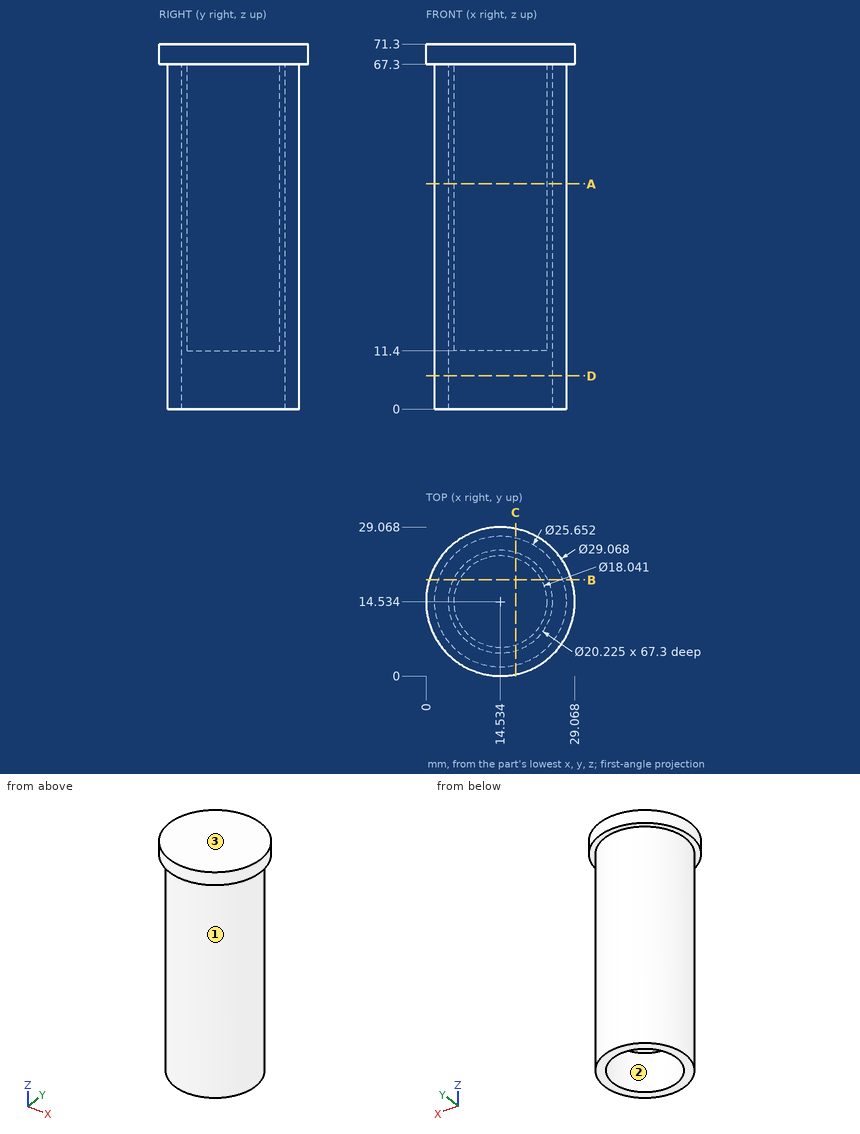
Design review of the part shown in the three views and the two pictorial views. Dimensions are in mm from the part's minimum x, y and z. Coordinates: 2 decimals unless noted, no trailing zeros. Order: outer loops, then holes, each group sorted by start corner. A loop starts at its lowest first (then second) coordinate and runs counter-clockwise, first axis right, second up. Notation, with made-up numbers: (38.5, 77) - (46.5, 77) arc R24 cw to (46.5, 91) - close; hole circle Ø6 at (5, -6). An arc over 180 degrees is marked (long way). Answer as CSV lines item,"result". Start each with the question number.
1) To check wall thickness, follow line 1 along X through (y, z) = (11.5, 13.5) (1 decimal); line 2 along Y through (x, z) = (16.25, 59) (1 decimal); line 3 along Y through (x, z) = (20.5, 53). State the ranges of each line that lie inside material, in increasing order. Write a range as [from, to].
2) Draft analysis for pull direction Y (two halves, no side actions). For the marked faces 1, 2 and 3, state which applies: +Y half, -Y half, draft (parallel to the pull), parting line (faces both ways), or undercut.
3) Add section C-C (x = 17.5). State the section outline as (y, z) points (1 decimal), then the cut area to 3 significant figures.
4) Add section D-D (z = 6.5). State the section outline as (x, y) points (1 decimal).
5) Add section A-A (z = 44). State the section outline as (x, y) points (1 decimal).
6) Add section B-B (y = 18.75). State the section outline as (x, z) points (1 decimal), then the cut area to 3 significant figures.
7) Insertion check: P1, Ø1, axis at x = 15, z = 31, coming from the +Y side; P2, Ø1.5, axis at x = 23, z = 52, coming from the +Y side; P3, Ø6, axis at x = 16.5, y = 10.5, coming from the -Z side. Each pin has a flat end and moves straight along its axis. Give the tip position at first contact, or say it passes through.
Result:
1,line 1,"[2.1, 4.9], [6, 23], [24.2, 27]"
1,line 2,"[1.8, 4.6], [5.7, 23.4], [24.5, 27.2]"
1,line 3,"[3.18, 6.37], [7.77, 21.3], [22.7, 25.89]"
2,face 1,"parting line"
2,face 2,"undercut"
2,face 3,"draft"
3,outline,"(0.3, 67.3) - (2.1, 67.3) - (2.1, 0) - (4.9, 0) - (4.9, 67.3) - (6, 67.3) - (6, 11.4) - (23.1, 11.4) - (23.1, 67.3) - (24.2, 67.3) - (24.2, 0) - (27, 0) - (27, 67.3) - (28.8, 67.3) - (28.8, 71.3) - (0.3, 71.3) - close"
3,area,"1,440 mm^2"
4,outline,"circle Ø25.7 at (14.5, 14.5); hole circle Ø20.2 at (14.5, 14.5)"
5,outline,"circle Ø25.7 at (14.5, 14.5); circle Ø18 at (14.5, 14.5); hole circle Ø20.2 at (14.5, 14.5)"
6,outline,"(0.6, 67.3) - (2.4, 67.3) - (2.4, 0) - (5.3, 0) - (5.3, 67.3) - (6.6, 67.3) - (6.6, 11.4) - (22.5, 11.4) - (22.5, 67.3) - (23.7, 67.3) - (23.7, 0) - (26.6, 0) - (26.6, 67.3) - (28.4, 67.3) - (28.4, 71.3) - (0.6, 71.3) - close"
6,area,"1,400 mm^2"
7,P1,"y = 27.36"
7,P2,"y = 24.78"
7,P3,"z = 11.4"
